Geometry: final body of the model. Coordinates: model frame, mm. A direction names the side the tool comes from. Coordinates: 2 decimals unless noted, no trailing zeros. Write each loop counter-clockwise with the first axis right and the second up, starting at its lowest first coordinate (ties: lowest second). Pieces come first, ordered by that corner, then holes.
from build123d import *

# Parameters (mm, degrees)
SKETCH1_W           = 42.299999982
SKETCH1_H           = 42.3
BOSS_EXTRUDE1_DEPTH = 38
CHAMFER1_SIZE       = 2.54
SKETCH2_R           = 11
BOSS_EXTRUDE2_DEPTH = 2
SKETCH3_R           = 2.25
BOSS_EXTRUDE3_DEPTH = 21
SKETCH4_W           = 3.436789712
SKETCH4_H           = 1.59509441
CUT_EXTRUDE1_DEPTH  = 18


with BuildPart() as part:
    # Sketch1 → Boss-Extrude1 (new body)
    with BuildSketch(Plane(origin=(0, 0, 0), x_dir=(1, 0, 0), z_dir=(0, 1, 0))):
        Rectangle(SKETCH1_W, SKETCH1_H)
    extrude(amount=BOSS_EXTRUDE1_DEPTH)

    # Chamfer1
    chamfer1_edges = [part.edges().sort_by_distance(p)[0] for p in [
        (21.149999991, 19, 21.15),
        (-21.149999991, 19, 21.15),
        (-21.149999991, 19, -21.15),
        (21.149999991, 19, -21.15),
    ]]
    chamfer(chamfer1_edges, length=CHAMFER1_SIZE)

    # Sketch2 → Boss-Extrude2 (add)
    with BuildSketch(Plane(origin=(0, 38, 0), x_dir=(1, 0, 0), z_dir=(0, 1, 0))):
        with Locations(Location((0, 0, 0), (0, 0, 270))):
            Circle(SKETCH2_R)
    extrude(amount=BOSS_EXTRUDE2_DEPTH)

    # Sketch3 → Boss-Extrude3 (add)
    with BuildSketch(Plane(origin=(0, 40, 0), x_dir=(1, 0, 0), z_dir=(0, 1, 0))):
        with Locations(Location((0, 0, 0), (0, 0, 90))):
            Circle(SKETCH3_R)
    extrude(amount=BOSS_EXTRUDE3_DEPTH)

    # Sketch4 → Cut-Extrude1 (cut)
    with BuildSketch(Plane(origin=(0, 61, 0), x_dir=(1, 0, 0), z_dir=(0, 1, 0))):
        with Locations((0, 2.25)):
            Rectangle(SKETCH4_W, SKETCH4_H)
    extrude(amount=-CUT_EXTRUDE1_DEPTH, mode=Mode.SUBTRACT)


solid = part.part
Item 1: Section A-A, the plane z = 0. Output: boundary loops of the cut face in (x, y).
Derived:
outline: (-21.15, 0) - (21.15, 0) - (21.15, 38) - (11, 38) - (11, 40) - (2.25, 40) - (2.25, 61) - (-2.25, 61) - (-2.25, 40) - (-11, 40) - (-11, 38) - (-21.15, 38) - close
Item 2: Section C-C, the plane y = 49. Output: boundary loops of the cut face in (x, z), plus the area to 3 significant figures.
Derived:
outline: (-1.72, -1.45) - (1.72, -1.45) arc R2.25 ccw (long way) to start
area: 14.0 mm2
Item 3: Material intervals for probe 1 along Y at (x, z) = (-13, 13.5); probe 2 along X at (y, z) = (52.5, -1), sorted ascending.
Derived:
probe 1: y = 0 to 38
probe 2: x = -2.02 to 2.02
Item 4: Section B-B, the plane x = 9. Output: boundary loops of the cut face in (y, z), plus the area to 3 significant figures.
Derived:
outline: (0, -21.15) - (38, -21.15) - (38, -6.32) - (40, -6.32) - (40, 6.32) - (38, 6.32) - (38, 21.15) - (0, 21.15) - close
area: 1,630 mm2
Item 5: Section D-D, the plane x = 0. Output: boundary loops of the cut face in (y, z), plus the area to 3 significant figures.
Derived:
outline: (0, -21.15) - (38, -21.15) - (38, -11) - (40, -11) - (40, -2.25) - (43, -2.25) - (43, -1.45) - (61, -1.45) - (61, 2.25) - (40, 2.25) - (40, 11) - (38, 11) - (38, 21.15) - (0, 21.15) - close
area: 1,730 mm2
Item 6: Set-up query: faces 1 (the flat face through (0, 52, -1.452)), 2 (the cylindrical face through (-0.099, 50.353, 2.248)), 3 (the flat face through (21.15, 19, 0)). Return all of +Z, -Z, +X, -X, +Y, -Y with unobstructed straight access to the full face (end or side cutting, diameter ignored); none if empty.
Derived:
face 1: -Z, +X, -X, +Y
face 2: +Y
face 3: +Z, -Z, +X, +Y, -Y
Item 7: Pin query (flat end, axial travel): pin 1 (0.6 mm diameter, centred on x = 1, z = -2, fed in from +Y); pin 2 (4 mm diameter, centred on x = -0.5, y = 51.5, fed in from -Z). Return the tip coordinate at first contact, or that it passes through.
Derived:
pin 1: stops at y = 43
pin 2: stops at z = -1.45
